For this review, take the finished solid that the model builds, in its own axes (mm). A direction names the side the tool comes from. Coordinates: 2 decimals unless noted, no trailing zeros. Loops run counter-clockwise (first coordinate to the right, second up) from the corner with the lowest first, then second, coordinate; pieces in that order, holes last. Notation, with made-up numbers: (53.5, 69.5) - (67.5, 69.5) arc R28 cw to (67.5, 89.5) - close; hole circle Ø5 at (23.5, 65). An arc over 180 degrees is marked (long way). One line per item, written item: value. Start each with the question number.
1. For faces 4 (the face through (1.639, -1.257, 11.259)), 5 (the face through (0, 1, 0)), 6 (the face through (-0.9, -1.4, 6.096)), list the 3-axis set-ups (+Z, -Z, +X, -X, +Y, -Y) from which the entire face can be reached by the end or side of a thin tool; tool diameter is ignored.
2. Take a section at D-D, the plane z = 2. State the section outline as (x, y) points.
3. Take a section at C-C, the plane z = 7.5. State the section outline as (x, y) points.
4. The part is to be moulded in two halves that separate along Y. For faces 1 (the face through (-0.743, 0.098, 7.138)), 2 (the face through (-1.43, 0.45, 3.01)), 3 (the face through (0.53, -1.32, 7.39)), say which applies: released by +Y, released by -Y, zero draft, split by the parting line, or undercut.
5. Take a section at B-B, the plane x = 0. State the section outline as (y, z) points, and give its area (3 significant figures).
6. Take a section at A-A, the plane y = 0. State the section outline as (x, z) points, and give its area (3 significant figures).
7. To check wall thickness, follow line 1 (Z direction, x = 0, y = 1.7); line 2 (X direction, y = 0, z = 7); line 3 (Z direction, x = -1.6, y = -0.3). State the ranges of each line that lie inside material, in increasing order. Write a range as from..to.
8. Insertion check: pin 1 (1.5 mm diameter, centred on x = 1.5, z = 6, fed in from -Y); pin 2 (2 mm diameter, centred on x = -0.5, z = 7.5, fed in from +Y). Each pin has a flat end and moves straight along its axis. Give the tip position at first contact, or say it passes through.
Autodesk Inventor part; units mm, degrees
ref_plane "YZ Plane" through (0, 0, 0) normal (1, 0, 0) x (0, 1, 0)
ref_plane "XY Plane" through (0, 0, 0) normal (0, 0, 1) x (1, 0, 0)
sketch "Sketch1" plane through (0, 0, 0) normal (0, 0, 1) x (1, 0, 0)
  circle A0 centre (0, 0) radius 2.159
  dimension "d0" = 4.318
extrude "Extrusion1" add sketch "Sketch1" along normal blind 8.128
sketch "Sketch2" plane through (0, 0, 0) normal (0, 0, -1) x (-1, 0, 0)
  circle A0 centre (0, 0) radius 2.159
  circle A1 centre (0, 0) radius 1.4986
  dimension "d3" = 2.9972
extrude "Extrusion2" cut sketch "Sketch2" against normal blind 6.096
sketch "Sketch3" plane through (0, 0, 0) normal (0, 1, 0) x (-1, 0, 0)
  line L0 (-2.159, 8.128) -> (2.159, 8.128)
  line L1 (0, -2.8448) -> (0, 17.0688)
  line L2 (2.159, 8.128) -> (0, 8.128)
  line L3 (0, 8.128) -> (0, 14.478)
  line L4 (2.159, 6.096) -> (-2.159, 6.096)
  line L5 (-2.159, 8.128) -> (2.159, 8.128)
  line L6 (2.159, 6.096) -> (2.159, 8.128)
  line L7 (-1.4986, 0) -> (1.4986, 0)
  line L8 (0, 14.478) -> (1.9685, 14.478)
  line L9 (1.9685, 14.478) -> (2.159, 8.128)
  point P0 (0, 0)
  dimension "d22" = 8.128
  dimension "d23" = 6.096
  dimension "d24" = 6.35
  dimension "d25" = 1.9685
revolve "Revolution1" add sketch "Sketch3" angle 360 about axis through (0, 0, -10) along (0, 0, 1) contours L1 L8 L9 L0
hole "Hole1" at (0, 0, 14.478) direction (0, 0, -1) diameter 1.4986 end through all
ref_plane "Work Plane1" through (0, 2.159, 0) normal (0, 1, 0) x (-1, 0, 0)
sketch "Sketch5" plane through (0, 2.159, 0) normal (0, 1, 0) x (-1, 0, 0)
  line L0 (2.159, 6.096) -> (-2.159, 6.096)
  line L1 (-2.159, 8.128) -> (2.159, 8.128)
  line L2 (0, -2.8956) -> (0, 17.3736)
  line L3 (0, 8.128) -> (0, 6.096)
  point P0 (0, 0)
  point P1 (0, 7.112)
hole "Hole2" at (0, 2.159, 7.112) direction (0, -1, 0) diameter 1.1938 end through all
equation "\"d25\" = 0.5 * d0 - 0.03 * d6"
properties part number "Tool_Mount_Luer_Adapter_Original" material "Acetal Resin, White"
Solutions:
1. face 4: +Z
1. face 5: -Z, +X, -X, +Y, -Y
1. face 6: -Z
2. outline: circle Ø3 at (0, 0); hole circle Ø1.5 at (0, 0)
3. outline: (-0.45, -2.11) - (-0.45, -0.6) arc R0.75 cw to (-0.45, 0.6) - (-0.45, 2.11) arc R2.16 ccw to start; (0.45, -2.11) arc R2.16 ccw to (0.45, 2.11) - (0.45, 0.6) arc R0.75 cw to (0.45, -0.6) - close
4. face 1: undercut
4. face 2: split by the parting line
4. face 3: zero draft
5. outline: (-2.16, 6.1) - (-1.5, 6.1) - (-1.5, 0) - (-0.75, 0) - (-0.75, 6.52) - (-2.16, 6.52) - close; (-2.16, 7.71) - (-0.75, 7.71) - (-0.75, 14.48) - (-1.97, 14.48) - (-2.16, 8.13) - close; (0.75, 0) - (1.5, 0) - (1.5, 6.1) - (2.16, 6.1) - (2.16, 6.52) - (0.75, 6.52) - close; (0.75, 7.71) - (2.16, 7.71) - (2.16, 8.13) - (1.97, 14.48) - (0.75, 14.48) - close
5. area: 28.2 mm2
6. outline: (-2.16, 6.1) - (-1.5, 6.1) - (-1.5, 0) - (-0.75, 0) - (-0.75, 14.48) - (-1.97, 14.48) - (-2.16, 8.13) - close; (0.75, 0) - (1.5, 0) - (1.5, 6.1) - (2.16, 6.1) - (2.16, 8.13) - (1.97, 14.48) - (0.75, 14.48) - close
6. area: 31.6 mm2
7. line 1: 6.1..6.52, 7.71..14.48
7. line 2: -2.16..-0.75, 0.75..2.16
7. line 3: 6.1..14.48
8. pin 1: y = -2.02
8. pin 2: y = 2.16
